Can you work these out from the model? Positions are in its coordinate system, mm. A direction names the side the tool comes from. Coordinates: 2 decimals unless noted, no trailing zeros. Order: outer loops, then holes, each group sorted by start corner. A loop starts at its lowest first (then second) coordinate and runs counter-clockwise, first axis right, second up.
```python
from build123d import *

# Parameters (mm, degrees)
SKETCH1_R           = 10
BOSS_EXTRUDE1_DEPTH = 335
SKETCH4_R           = 7.5
BOSS_EXTRUDE2_DEPTH = 40
SKETCH5_R           = 6
BOSS_EXTRUDE3_DEPTH = 12
BOSS_EXTRUDE5_START = 50
SKETCH11_R          = 7.5
BOSS_EXTRUDE5_DEPTH = 50
CHAMFER2_SIZE       = 0.5


with BuildPart() as part:
    # Sketch1 → Boss-Extrude1 (new, symmetric)
    with BuildSketch(Plane.XY):
        Circle(SKETCH1_R)
    extrude(amount=BOSS_EXTRUDE1_DEPTH, both=True)

    # Sketch4 → Boss-Extrude2 (add)
    with BuildSketch(Plane.XY.offset(335)):
        Circle(SKETCH4_R)
    extrude(amount=BOSS_EXTRUDE2_DEPTH)

    # Sketch5 → Boss-Extrude3 (add)
    with BuildSketch(Plane.XY.offset(375)):
        Circle(SKETCH5_R)
    extrude(amount=BOSS_EXTRUDE3_DEPTH)

    # Sketch11 → Boss-Extrude5 (add)
    with BuildSketch(Plane(origin=(0, 0, -335), x_dir=(-1, 0, 0), z_dir=(0, 0, -1)).offset(BOSS_EXTRUDE5_START)):
        with Locations(Location((0, 0, 0), (0, 0, 180))):
            Circle(SKETCH11_R)
    extrude(amount=-BOSS_EXTRUDE5_DEPTH)

    # Chamfer2
    chamfer2_edges = [part.edges().sort_by_distance(p)[0] for p in [
        (-6, 0, 387),
        (-7.5, 0, -385),
        (-10, 0, -335),
        (-10, 0, 335),
        (-7.5, 0, 375),
    ]]
    chamfer(chamfer2_edges, length=CHAMFER2_SIZE)


solid = part.part
```
1. I'm going to push flat-ended pins straight in: pin 1 (4 mm diameter, centred on x = 4.5, z = 197, fed in from -Y); pin 2 (8 mm diameter, centred on y = 5.5, z = 204.5, fed in from +X); pin 3 (2 mm diameter, centred on y = 3.5, z = -249, fed in from +X). Where does each tip first touch, or does it pass through?
Completed:
pin 1: stops at y = -9.68
pin 2: stops at x = 9.89
pin 3: stops at x = 9.68
2. Please list where these lines run through material, in increasing order: probe 1 along Z at (x, y) = (6, -3); probe 2 along Y at (x, z) = (1.5, -90); probe 3 along Z at (x, y) = (7.5, -5).
Completed:
probe 1: z = -385 to 375
probe 2: y = -9.89 to 9.89
probe 3: z = -335 to 335
3. Imagine slicing it at C-C on z = 60.5. Please give me the cut outline in (x, y).
Completed:
outline: circle Ø20 at (0, 0)
4. On a 3-axis mill with a long thin cutter (end or side, diameter ignored), from which of +Z, -Z, +X, -X, +Y, -Y can I reach the whole of each face in a straight line? I mean faces 1 (the cylindrical face through (4.032, -6.324, -360.096)), 2 (the cylindrical face through (-2.17, -9.76, 4.68)), 3 (the cylindrical face through (-7.493, 0.33, 354.474)). Say none if no direction works.
Completed:
face 1: -Z
face 2: +Z, -Z
face 3: +Z
5. Imagine slicing it at A-A on x = 0. Please give me the cut outline in (y, z), then the cut area to 3 significant figures.
Completed:
outline: (-10, -334.5) - (-9.5, -335) - (-7.5, -335) - (-7.5, -384.5) - (-7, -385) - (7, -385) - (7.5, -384.5) - (7.5, -335) - (9.5, -335) - (10, -334.5) - (10, 334.5) - (9.5, 335) - (7.5, 335) - (7.5, 374.5) - (7, 375) - (6, 375) - (6, 386.5) - (5.5, 387) - (-5.5, 387) - (-6, 386.5) - (-6, 375) - (-7, 375) - (-7.5, 374.5) - (-7.5, 335) - (-9.5, 335) - (-10, 334.5) - close
area: 14,900 mm2
